from build123d import *

# Parameters (mm, degrees)
ESQUISSE1_W             = 32
ESQUISSE1_H             = 32
BOSS_EXTRU_1_DEPTH      = 2.2
ESQUISSE2_R             = 3.5
BOSS_EXTRU_2_DEPTH      = 33
ESQUISSE3_R             = 3
ENL_V_MAT_EXTRU_1_DEPTH = 44.447262572


with BuildPart() as part:
    # Esquisse1 → Boss.-Extru.1 (new body)
    with BuildSketch(Plane.XY):
        with Locations((-1.848605578, 2.167330677)):
            Rectangle(ESQUISSE1_W, ESQUISSE1_H)
    extrude(amount=BOSS_EXTRU_1_DEPTH)

    # Esquisse2 → Boss.-Extru.2 (add)
    with BuildSketch(Plane.XY.offset(2.2)):
        with Locations((-1.848605578, 2.167330677)):
            Circle(ESQUISSE2_R)
    extrude(amount=BOSS_EXTRU_2_DEPTH)

    # Esquisse3 → Enlèv. mat.-Extru.1 (cut, through all)
    with BuildSketch(Plane.XY.offset(35.2)):
        with Locations((-1.848605578, 2.167330677)):
            Circle(ESQUISSE3_R)
    extrude(amount=-ENL_V_MAT_EXTRU_1_DEPTH, mode=Mode.SUBTRACT)


solid = part.part
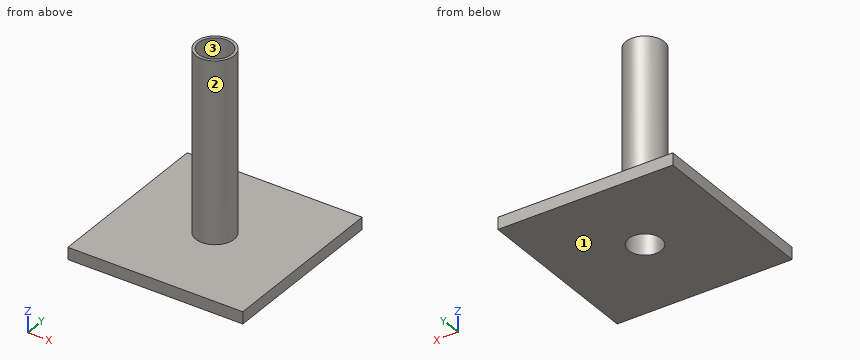
The listing builds one solid part. Answer for the finished solid, in the listing's coordinates (mm). Face numbers are marked on the shaded views. Give positions to 0.01 mm unless a question says otherwise; leave off trailing zeros. Order: outer loops, then holes, each group sorted by start corner. A loop starts at its lowest first (then second) coordinate and runs counter-clockwise, first axis right, second up. Notation, with made-up numbers: (59, 39.25) - (89, 39.25) arc R20 cw to (89, 76.25) - close; hole circle Ø11 at (16, 81.25). An arc over 180 degrees is marked (long way). One line per item, written item: value. Start each with the question number.
1) A cutting plane is placed at D-D on x = 6. Give the vertices of the cut face in (y, z).
2) A cutting plane is placed at A-A on x = -3. Give the vertices of the cut face in (y, z), then the cut area to 3 significant figures.
3) Given pin 1 Ø8 at (x, z) = (4, 13) entering from -Y; pin 2 Ø9.5 at (x, y) = (-4, 9.5) entering from +Z; pin 3 Ø12 at (y, z) = (3, 22) entering from -X; pin 4 Ø4 at (x, z) = (-3, 24) entering from -Y, each flat-ended and moving along its own axis, determine where each tip first touches the part or whether it passes through.
4) A cutting plane is placed at B-B on y = 4. Give the vertices of the cut face in (x, z).
5) The mould has two halves that part along X. Classify the marked faces 1, 2 and 3: released by +X, released by -X, zero draft, split by the parting line, or undercut.
6) Find the intervals of material crossed by L1, parallel to Z at x = -8.5, y = -9; L2, parallel to X at y = 2.5, z = 16; L3, parallel to X at y = 4, z = 17, in increasing order.
7) A cutting plane is placed at C-C on z = 23.5. Give the vertices of the cut face in (x, y).
Answer sheet:
1. outline: (-13.83, 0) - (18.17, 0) - (18.17, 2.2) - (-13.83, 2.2) - close
2. outline: (-13.83, 0) - (-0.6, 0) - (-0.6, 35.2) - (-1.14, 35.2) - (-1.14, 2.2) - (-13.83, 2.2) - close; (4.94, 0) - (18.17, 0) - (18.17, 2.2) - (5.47, 2.2) - (5.47, 35.2) - (4.94, 35.2) - close
2. area: 93.5 mm2
3. pin 1: stops at y = -0.8
3. pin 2: stops at z = 35.2
3. pin 3: stops at x = -5.35
3. pin 4: stops at y = -1.33
4. outline: (-17.85, 0) - (-4.22, 0) - (-4.22, 35.2) - (-4.83, 35.2) - (-4.83, 2.2) - (-17.85, 2.2) - close; (0.53, 0) - (14.15, 0) - (14.15, 2.2) - (1.13, 2.2) - (1.13, 35.2) - (0.53, 35.2) - close
5. face 1: zero draft
5. face 2: split by the parting line
5. face 3: undercut
6. L1: z = 0 to 2.2
6. L2: x = -5.33 to -4.83, 1.13 to 1.64
6. L3: x = -4.83 to -4.22, 0.53 to 1.13
7. outline: circle Ø7 at (-1.85, 2.17); hole circle Ø6 at (-1.85, 2.17)
